Input: part model. Units: mm. Frame: model coordinates. Face numbers are marked on the shaded views. A direction names the side the tool comes from. Give positions to 0.01 mm unless a question says otherwise; leave off trailing zeros. Loops run counter-clockwise (first coordinate to the right, second up) from the corner with the lowest first, then second, coordinate; pieces in that order, holes last. Notation, with made-up numbers: (-28.5, 17.25) - (-0.5, 17.25) arc R13 ccw to (-0.5, 42.25) - close; hole circle Ø8 at (-15, 31). An arc over 180 degrees is marked (long way). One line per item, written item: value.
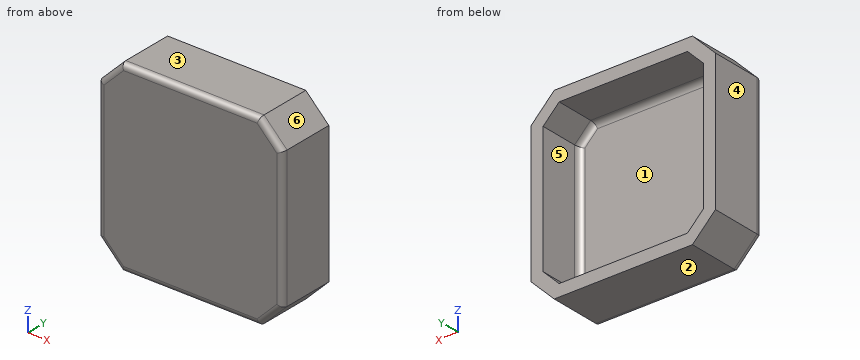
from build123d import *

# Parameters (mm, degrees)
SKETCH1_W      = 65
SKETCH1_H      = 65
EXTRUDE1_DEPTH = 4.4
CHAMFER1_SIZE  = 8.125
EXTRUDE2_DEPTH = 15.6
FILLET1_R      = 2


with BuildPart() as part:
    # Sketch1 → Extrude1 (new body)
    with BuildSketch(Plane(origin=(0, 0, 0), x_dir=(1, 0, 0), z_dir=(0, 1, 0))):
        Rectangle(SKETCH1_W, SKETCH1_H)
    extrude(amount=EXTRUDE1_DEPTH)

    # Chamfer1
    chamfer1_edges = [part.edges().sort_by_distance(p)[0] for p in [
        (32.5, 2.2, 32.5),
        (-32.5, 2.2, 32.5),
        (-32.5, 2.2, -32.5),
        (32.5, 2.2, -32.5),
    ]]
    chamfer(chamfer1_edges, length=CHAMFER1_SIZE)

    # Sketch2 → Extrude2 (add)
    with BuildSketch(Plane(origin=(0, 4.4, 0), x_dir=(1, 0, 0), z_dir=(0, 1, 0))):
        Polygon((32.5, 24.375), (24.375, 32.5), (-24.375, 32.5), (-32.5, 24.375), (-32.5, -24.375), (-24.375, -32.5), (24.375, -32.5), (32.5, -24.375), align=None)
        Polygon((-22.635303038, 28.3), (-28.3, 22.635303038), (-28.3, -22.635303038), (-22.635303038, -28.3), (15.182932057, -28.3), (22.635303038, -28.3), (28.3, -22.635303038), (28.3, 22.635303038), (22.635303038, 28.3), align=None, mode=Mode.SUBTRACT)
    extrude(amount=EXTRUDE2_DEPTH)

    # Fillet1
    fillet1_edges = [part.edges().sort_by_distance(p)[0] for p in [
        (-32.5, 0, 0),
        (32.5, 0, 0),
        (0, 0, 32.5),
        (0, 0, -32.5),
        (-28.4375, 0, 28.4375),
        (28.4375, 0, 28.4375),
        (28.4375, 0, -28.4375),
        (-28.4375, 0, -28.4375),
        (-25.467651519, 4.4, -25.467651519),
        (-28.3, 4.4, 0),
        (-25.467651519, 4.4, 25.467651519),
        (0, 4.4, 28.3),
        (25.467651519, 4.4, 25.467651519),
        (28.3, 4.4, 0),
        (25.467651519, 4.4, -25.467651519),
        (0, 4.4, -28.3),
    ]]
    fillet(fillet1_edges, radius=FILLET1_R)


solid = part.part
Item 1: Access query for the marked faces 1 and 2. Directions: +Z, -Z, +X, -X, +Y, -Y. A direction counts if a zero-diameter tool reaches every point of the face in a straight line with its end or side. Return the directions, or none.
Verdict:
face 1: +Y
face 2: -Z, +X, -X, +Y, -Y
Item 2: Section D-D, the plane z = -17.5. Output: boundary loops of the cut face in (x, y).
Verdict:
outline: (-32.5, 2) arc R2 ccw to (-30.5, 0) - (30.5, 0) arc R2 ccw to (32.5, 2) - (32.5, 20) - (28.3, 20) - (28.3, 6.4) arc R2 cw to (26.3, 4.4) - (-26.3, 4.4) arc R2 cw to (-28.3, 6.4) - (-28.3, 20) - (-32.5, 20) - close
Item 3: Pin query (flat end, axial travel): P1, Ø8, axis at x = -7.5, z = -24, coming from the +Y side. Return the tip coordinate at first contact, or that it passes through.
Verdict:
P1: stops at y = 5.35
Item 4: Section B-B, the plane x = -21. Output: boundary loops of the cut face in (y, z).
Verdict:
outline: (0, -30.5) arc R2 ccw to (2, -32.5) - (20, -32.5) - (20, -28.3) - (6.4, -28.3) arc R2 cw to (4.4, -26.3) - (4.4, 26.3) arc R2 cw to (6.4, 28.3) - (20, 28.3) - (20, 32.5) - (2, 32.5) arc R2 ccw to (0, 30.5) - close
Item 5: Section A-A, the plane y = 3. Output: boundary loops of the cut face in (x, z) (3 decimals), and give its area (3 significant figures).
Verdict:
outline: (-32.5, -24.375) - (-24.375, -32.5) - (24.375, -32.5) - (32.5, -24.375) - (32.5, 24.375) - (24.375, 32.5) - (-24.375, 32.5) - (-32.5, 24.375) - close
area: 4,090 mm^2
Item 6: Section C-C, the plane y = 15.75. Output: boundary loops of the cut face in (x, z) (3 decimals).
Verdict:
outline: (-32.5, -24.375) - (-24.375, -32.5) - (24.375, -32.5) - (32.5, -24.375) - (32.5, 24.375) - (24.375, 32.5) - (-24.375, 32.5) - (-32.5, 24.375) - close; hole (-28.3, -22.635) - (-22.635, -28.3) - (22.635, -28.3) - (28.3, -22.635) - (28.3, 22.635) - (22.635, 28.3) - (-22.635, 28.3) - (-28.3, 22.635) - close
Item 7: Draft query along X for the marked faces 3, 4, 5 and 6. Return one class per face: pulls with the +X half, pulls with the -X half, needs draft (parallel to the pull), parting line crosses it, or undercut.
Verdict:
face 3: needs draft
face 4: pulls with the -X half
face 5: undercut
face 6: pulls with the +X half
Item 8: Material intervals for L1, parallel to Z at x = 15.5, y = 15; L2, parallel to Y at x = 22, z = -23, sorted ascending.
Verdict:
L1: z = -32.5 to -28.3, 28.3 to 32.5
L2: y = 0 to 4.4
